Source: CAD feature listing. Evaluate the final solid. Frame: model axes, mm. A direction names the side the tool comes from. Round coordinates to 2 decimals unless told otherwise and drop trailing zeros. Order: outer loops, then holes, each group sorted by start corner. A loop starts at its lowest first (then second) coordinate and runs counter-clockwise, first axis right, second up. Notation, with made-up numbers: (50, -7.5) - (83, -7.5) arc R22 cw to (83, 1.5) - close; hole circle Ø9 at (-28.5, 38). An arc over 180 degrees is marked (long way). Use one line per item in the form item = value. Start each with the question number.
Q1. Cut plane A-A, the plane y = -50. Return the cut outline in (x, z).
Q2. Ray query, line 1 (Y direction, x = 35, z = 7.5); line 2 (X direction, y = 3, z = 32.5); line 3 (Z direction, x = 53, y = 1.5). Return the intervals inside material, ascending. Write a range as [from, to].
Q3. Draft query along X for faces 1 (the cylindrical face through (34.288, 77.683, 60.03)), 2 (the cylindrical face through (-6.65, -5.26, 33.01)), 3 (the flat face through (34, 34, 0)). Return one class per face: released by +X, released by -X, zero draft, split by the parting line, or undercut.
Q4. Cut plane B-B, the plane z = 39. Return the cut outline in (x, y).
Q5. Pin query (flat end, axial travel): pin 1 Ø1.8 at (x, y) = (35, 28.2) entering from +Z; pin 2 Ø10 at (y, z) = (28, 9) entering from -X; pin 3 Ø12.5 at (x, y) = (35, 20.6) entering from +Z. Return the tip coordinate at first contact, or that it passes through.
Q6. Cut plane C-C, the plane x = 69. Return the cut outline in (y, z), and give its area (3 significant figures).
Q7. Set-up query: faces 4 (the cylindrical face through (19.673, -55.153, 62.142)), 5 (the flat face through (34, -58, 62)), 6 (the flat face through (34, -29, 59.1)), 7 (the cylindrical face through (78.214, -2.55, 33.006)). Return all of +Z, -Z, +X, -X, +Y, -Y with unobstructed straight access to the full face (end or side cutting, diameter ignored); none if empty.
Autodesk Inventor part; units mm, degrees
ref_plane "YZ Plane" through (0, 0, 0) normal (1, 0, 0) x (0, 1, 0)
ref_plane "XZ Plane" through (0, 0, 0) normal (0, 1, 0) x (-1, 0, 0)
ref_plane "XY Plane" through (0, 0, 0) normal (0, 0, 1) x (1, 0, 0)
sketch "Sketch1" plane through (0, 0, 0) normal (0, 0, 1) x (1, 0, 0)
  line L0 (0, 0) -> (70, 0)
  line L1 (70, 0) -> (35, 60.6218)
  line L2 (35, 60.6218) -> (0, 0)
  circle A0 centre (35, 20.5961) radius 5.5
  circle A1 centre (35, 57.6961) radius 20
  point P0 (46.2401, 41.1534)
  point P1 (23.7599, 41.1534)
  dimension "d0" = 70
  dimension "d1" = 70
  dimension "d2" = 60
  dimension "d3" = 11
  dimension "d4" = 37.1
  dimension "d5" = 40
extrude "Extrusion1" add sketch "Sketch1" along normal blind 65.1
ref_plane "Work Plane1" through (0, 0, 55.1) normal (0, 0, 1) x (1, 0, 0)
sketch "Sketch2" plane through (0, 0, 55.1) normal (0, 0, 1) x (1, 0, 0)
  line L0 (14.3119, 82.6705) -> (-13.7787, 82.6705)
  line L1 (-13.7787, 82.6705) -> (-13.7787, -9.2093)
  line L2 (-13.7787, -9.2093) -> (82.9291, -9.2093)
  line L3 (82.9291, -9.2093) -> (82.9291, 82.6705)
  line L4 (82.9291, 82.6705) -> (14.3119, 82.6705)
  point P0 (0, 0)
extrude "Extrusion2" cut sketch "Sketch2" against normal blind 45.2
sketch "Sketch3" plane through (0, 0, 65.1) normal (0, 0, 1) x (1, 0, 0)
  arc A0 (46.2401, 41.1534) -> (23.7599, 41.1534) centre (35, 57.6961) ccw
  circle A1 centre (35, 57.6961) radius 4.5
  point P0 (0, 0)
  dimension "d11" = 9
extrude "Extrusion3" cut sketch "Sketch3" against normal through all
pattern_circular "Circular Pattern1" count 3 over 360 about axis through (35, 20.5961, 0) along (0, 0, 1) of "Extrusion3"
sketch "Sketch4" plane through (0, 0, 65.1) normal (0, 0, 1) x (1, 0, 0)
  arc A0 (6.8784, 0) -> (3.7314, 6.463) centre (2.8705, 2.0461) ccw
  circle A1 centre (2.8705, 2.0461) radius 4.5
  circle A2 centre (2.8705, 2.0461) radius 12
  arc A3 (66.2686, 6.463) -> (63.1216, 0) centre (67.1295, 2.0461) ccw
  circle A4 centre (67.1295, 2.0461) radius 4.5
  circle A5 centre (67.1295, 2.0461) radius 12
  point P0 (0, 0)
  point P1 (63.1216, 0)
  point P2 (66.2686, 6.463)
  point P3 (6.8784, 0)
  point P4 (3.7314, 6.463)
  dimension "d17" = 24
  dimension "d18" = 24
extrude "Extrusion4" add sketch "Sketch4" against normal blind 65.1
sketch "Sketch5" plane through (0, 0, 65.1) normal (0, 0, 1) x (1, 0, 0)
  line L0 (23.7599, 41.1534) -> (7.5589, 13.0923)
  line L1 (13.3053, -58) -> (55.3053, -58)
  line L2 (55.3053, -58) -> (55.3053, 0)
  line L3 (14.6947, 0) -> (55.3053, 0)
  line L4 (13.3053, -58) -> (13.3053, 0)
  line L5 (13.3053, 0) -> (15.6594, 0)
  point P0 (0, 0)
  dimension "d22" = 42
  dimension "d24" = 0
  dimension "d26" = 58
extrude "Extrusion5" add sketch "Sketch5" against normal blind 6
sketch "Sketch6" plane through (0, 0, 65.1) normal (0, 0, 1) x (1, 0, 0)
  circle A0 centre (35, 20.5961) radius 5.5
  circle A1 centre (35, 20.5961) radius 11
  point P0 (0, 0)
  dimension "d29" = 22
extrude "Extrusion6" cut sketch "Sketch6" against normal blind 8
sketch "Sketch7" plane through (35, 20.5961, 57.1) normal (0, 0, 1) x (1, 0, 0)
  circle A0 centre (-0.0422, -7.6) radius 1.25
  circle A1 centre (0, 0) radius 5.5
  point P0 (-35, -20.5961)
  dimension "d32" = 2.5
  dimension "d33" = 7.6
extrude "Extrusion7" cut sketch "Sketch7" against normal blind 5 contours A0
sketch "Sketch8" plane through (0, 0, 65.1) normal (0, 0, 1) x (1, 0, 0)
  line L0 (18.1078, -53.5536) -> (18.1078, -11.6696)
  line L1 (18.1078, -11.6696) -> (21.3078, -11.6696)
  line L2 (21.3078, -11.6696) -> (21.3078, -53.5536)
  line L3 (21.3078, -53.5536) -> (18.1078, -53.5536)
  line L4 (51.8078, -11.6696) -> (51.8078, -53.5536)
  line L5 (51.8078, -53.5536) -> (48.6078, -53.5536)
  line L6 (48.6078, -53.5536) -> (48.6078, -11.6696)
  line L7 (48.6078, -11.6696) -> (51.8078, -11.6696)
  circle A0 centre (34.9578, 12.9961) radius 1.25
  arc A1 (48.6078, -53.5536) -> (51.8078, -53.5536) centre (50.2078, -53.5536) ccw
  arc A2 (51.8078, -11.6696) -> (48.6078, -11.6696) centre (50.2078, -11.6696) ccw
  arc A3 (18.1078, -53.5536) -> (21.3078, -53.5536) centre (19.7078, -53.5536) ccw
  arc A4 (21.3078, -11.6696) -> (18.1078, -11.6696) centre (19.7078, -11.6696) ccw
  point P0 (0, 0)
  point P1 (21.7083, -32.6116)
  point P2 (52.2083, -32.6116)
  dimension "d36" = 3.2
  dimension "d37" = 3.2
  dimension "d38" = 30.5
  dimension "d41" = 13.65
  dimension "d42" = 13.65
extrude "Extrusion8" cut sketch "Sketch8" against normal blind 10 contours L0 L1 L2 L3 | L3 A3 | A4 L1 | L4 L5 L6 L7 | L7 A2 | A1 L5
sketch "Sketch9" plane through (0, 0, 65.1) normal (0, 0, 1) x (1, 0, 0)
  circle A0 centre (35, 28.1961) radius 1.1
  circle A1 centre (35, 20.5961) radius 5.5
  point P0 (0, 0)
  dimension "d45" = 2.2
  dimension "d46" = 7.6
extrude "Extrusion9" cut sketch "Sketch9" against normal blind 10 contours A0
sketch "Sketch10" plane through (0, 0, 65.1) normal (0, 0, 1) x (1, 0, 0)
  circle A0 centre (35, 35.2401) radius 2.5
  point P0 (0, 0)
  dimension "d49" = 5
extrude "Extrusion10" add sketch "Sketch10" against normal blind 65
properties part number "Platform 1 piece"
Completed:
q1.outline = (13.31, 59.1) - (18.11, 59.1) - (18.11, 65.1) - (13.31, 65.1) - close; (21.31, 59.1) - (48.61, 59.1) - (48.61, 65.1) - (21.31, 65.1) - close; (51.81, 59.1) - (55.31, 59.1) - (55.31, 65.1) - (51.81, 65.1) - close
q2.line_1 = [0, 15.1], [26.1, 53.2], [62.2, 77.7]
q2.line_2 = [-9.09, -1.53], [7.27, 14.83], [55.17, 62.73], [71.53, 79.09]
q2.line_3 = [0, 9.9], [55.1, 65.1]
q3.face_1 = split by the parting line
q3.face_2 = undercut
q3.face_3 = zero draft
q4.outline = circle Ø24 at (2.87, 2.05); circle Ø5 at (35, 35.24); circle Ø24 at (67.13, 2.05); hole (3.73, 6.46) arc R4.5 ccw (long way) to (6.88, 0) arc R4.5 ccw to start; hole (63.12, 0) arc R4.5 ccw (long way) to (66.27, 6.46) arc R4.5 ccw to start
q5.pin_1 = 9.9
q5.pin_2 = 13.28
q5.pin_3 = 57.1
q6.outline = (-9.81, 0) - (-2.05, 0) - (-2.05, 65.1) - (-9.81, 65.1) - close; (6.14, 0) - (13.9, 0) - (13.9, 65.1) - (6.14, 65.1) - close
q6.area = 1,010 mm2
q7.face_4 = +Z, -Z
q7.face_5 = +Z, -Z, +X, -X, -Y
q7.face_6 = -Z, -Y
q7.face_7 = none
